Geometry: final body of the model. Coordinates: model frame, mm. A direction names the side the tool comes from. Give positions to 0.01 mm unless a question says otherwise; leave off trailing zeros. Loops run counter-clockwise (first coordinate to the right, second up) from the corner with the lowest first, then second, coordinate; pieces in that order, holes last.
```python
from build123d import *

# Parameters (mm, degrees)
SKETCH2_W            = 120.65
SKETCH2_H            = 50.8
BOSS_EXTRUDE1_DEPTH  = 6.35
SKETCH3_R            = 14.2875
CUT_EXTRUDE1_DEPTH   = 6.35
SKETCH6_W            = 38.1
SKETCH6_H            = 19.05
BOSS_EXTRUDE2_DEPTH  = 6.35
FILLET2_R            = 6.35
FILLET1_R            = 2.54
SKETCH8_W            = 50.8
SKETCH8_H            = 63.5
BOSS_EXTRUDE3_DEPTH  = 6.35
FILLET3_R            = 12.7
SKETCH9_R            = 3.175
CUT_EXTRUDE2_DEPTH   = 6.35
LPATTERN1_COUNT      = 3
LPATTERN1_PITCH      = 19.05
LPATTERN1_COUNT_DIR2 = 2
LPATTERN1_PITCH_DIR2 = 19.05


with BuildPart() as part:
    # Sketch2 → Boss-Extrude1 (new body)
    with BuildSketch(Plane(origin=(0, 0, 0), x_dir=(1, 0, 0), z_dir=(0, 1, 0))):
        with Locations((7.924270833, 15.531041667)):
            Rectangle(SKETCH2_W, SKETCH2_H)
    extrude(amount=BOSS_EXTRUDE1_DEPTH)

    # Sketch3 → Cut-Extrude1 (cut)
    with BuildSketch(Plane(origin=(0, 6.35, 0), x_dir=(1, 0, 0), z_dir=(0, 1, 0))):
        with Locations(Location((-32.715729167, 15.61478805, 0), (0, 0, 270))):
            Circle(SKETCH3_R)
    cut_extrude1 = extrude(amount=-CUT_EXTRUDE1_DEPTH, mode=Mode.SUBTRACT)

    # Mirror1: Cut-Extrude1 across plane
    add(cut_extrude1.mirror(Plane(origin=(7.924270833, 0, 0), x_dir=(0, 0, 1), z_dir=(1, 0, 0))), mode=Mode.SUBTRACT)

    # Sketch6 → Boss-Extrude2 (add)
    with BuildSketch(Plane(origin=(0, 6.35, 0), x_dir=(1, 0, 0), z_dir=(0, 1, 0))):
        with Locations((-71.450729167, -0.343958333)):
            Rectangle(SKETCH6_W, SKETCH6_H)
    boss_extrude2 = extrude(amount=-BOSS_EXTRUDE2_DEPTH)

    # Mirror2: Boss-Extrude2 across plane
    add(boss_extrude2.mirror(Plane(origin=(7.924270833, 0, 0), x_dir=(0, 0, 1), z_dir=(1, 0, 0))))

    # Fillet2
    fillet2_edges = [part.edges().sort_by_distance(p)[0] for p in [
        (-52.400729167, 3.175, -9.181041667),
        (68.249270833, 3.175, -9.181041667),
    ]]
    fillet(fillet2_edges, radius=FILLET2_R)

    # Fillet1
    fillet1_edges = [part.edges().sort_by_distance(p)[0] for p in [
        (-90.500729167, 3.175, 9.868958333),
        (-90.500729167, 3.175, -9.181041667),
        (106.349270833, 3.175, -9.181041667),
        (106.349270833, 3.175, 9.868958333),
        (-52.400729167, 3.175, -40.931041667),
        (68.249270833, 3.175, -40.931041667),
    ]]
    fillet(fillet1_edges, radius=FILLET1_R)

    # Sketch8 → Boss-Extrude3 (add)
    with BuildSketch(Plane(origin=(0, 6.35, 0), x_dir=(1, 0, 0), z_dir=(0, 1, 0))):
        with Locations((10.464270833, -41.618958333)):
            Rectangle(SKETCH8_W, SKETCH8_H)
    extrude(amount=-BOSS_EXTRUDE3_DEPTH)

    # Fillet3
    fillet3_edges = [part.edges().sort_by_distance(p)[0] for p in [
        (-14.935729167, 3.175, 9.868958333),
        (35.864270833, 3.175, 9.868958333),
    ]]
    fillet(fillet3_edges, radius=FILLET3_R)

    # Sketch9 → Cut-Extrude2 (cut)
    with BuildSketch(Plane(origin=(0, 6.35, 0), x_dir=(1, 0, 0), z_dir=(0, 1, 0))):
        with Locations(Location((-8.585729167, -54.318958333, 0), (0, 0, 270))):
            Circle(SKETCH9_R)
    cut_extrude2 = extrude(amount=-CUT_EXTRUDE2_DEPTH, mode=Mode.SUBTRACT)

    # LPattern1: Cut-Extrude2 3 × 2
    with Locations(*[(i * LPATTERN1_PITCH, 0, -j * LPATTERN1_PITCH_DIR2) for i in range(LPATTERN1_COUNT) for j in range(LPATTERN1_COUNT_DIR2) if (i, j) != (0, 0)]):
        add(cut_extrude2, mode=Mode.SUBTRACT)


solid = part.part
```
Q1. Section query C-C, the plane x = -44.5. Return loops of the section in (y, z).
Q2. Section query B-B, the plane z = -23. Return loops of the section in (x, y), and give its area (3 significant figures).
Q3. Reachability of faces 1 (the face through (-57, 3, 9.869)), 2 (the face through (68.249, 3, -27)), 3 (the face through (-52.401, 3, -27)), 4 (the face through (77, 3, 9.869)), 5 (the face through (9, 6.35, 3)) from +Z, -Z, +X, -X, +Y, -Y: full face, straight path, thin tool, end or side. Return the list, or none.
Q4. Section query A-A, the plane y = 2. State how many separate pieces and enclosed holes the cut face has, and give its area (3 significant figures).
Q5. Pin query (flat end, axial travel): pin 1 Ø1.9 at (y, z) = (2.5, -27.5) entering from -X; pin 2 Ø5.5 at (x, z) = (10.46, 35.27) entering from +Y; pin 3 Ø1.9 at (y, z) = (3, -32.5) entering from +X; pin 4 Ø1.5 at (y, z) = (4, -12) entering from -X. Return the tip coordinate at first contact, or that it passes through.
Q6. Section query D-D, the plane z = 62.5. Return loops of the section in (x, y).
Q7. Mould query, pull axis Z, two halves, no side actions, for faces 6 (the face through (106.349, 3, 0)), 7 (the face through (61.24, 3.22, -9.02)), 8 (the face through (-74, 3, -9.181)). Classes: +Z half, -Z half, draft (parallel to the pull), parting line (faces both ways), or undercut.
Q8. Material intervals for probe 1 along X at (y, z) = (3.75, 54); probe 2 along X at (y, z) = (2, -13.5); probe 3 along X at (y, z) = (4.25, -18), sorted ascending.
Resolved:
1. outline: (0, -40.93) - (6.35, -40.93) - (6.35, -23.69) - (0, -23.69) - close; (0, -7.54) - (6.35, -7.54) - (6.35, 9.87) - (0, 9.87) - close
2. outline: (-52.4, 0) - (-44.95, 0) - (-44.95, 6.35) - (-52.4, 6.35) - close; (-20.48, 0) - (36.33, 0) - (36.33, 6.35) - (-20.48, 6.35) - close; (60.8, 0) - (68.25, 0) - (68.25, 6.35) - (60.8, 6.35) - close
2. area: 455 mm2
3. face 1: +Z, -X, +Y, -Y
3. face 2: -Z, +X, +Y, -Y
3. face 3: -Z, -X, +Y, -Y
3. face 4: +Z, +X, +Y, -Y
3. face 5: +Z, -Z, +X, -X, +Y
4. separate pieces: 1
4. enclosed holes: 8
4. area: 9,410 mm2
5. pin 1: stops at x = -52.4
5. pin 2: passes through
5. pin 3: stops at x = 68.25
5. pin 4: stops at x = -54.06
6. outline: (-14.94, 0) - (35.86, 0) - (35.86, 6.35) - (-14.94, 6.35) - close
7. face 6: draft
7. face 7: undercut
7. face 8: -Z half
8. probe 1: x = -14.94 to -11.74, -5.43 to 7.31, 13.62 to 26.36, 32.67 to 35.86
8. probe 2: x = -52.73 to -46.85, -18.59 to 34.43, 62.69 to 68.58
8. probe 3: x = -52.4 to -46.8, -18.63 to 34.48, 62.65 to 68.25
